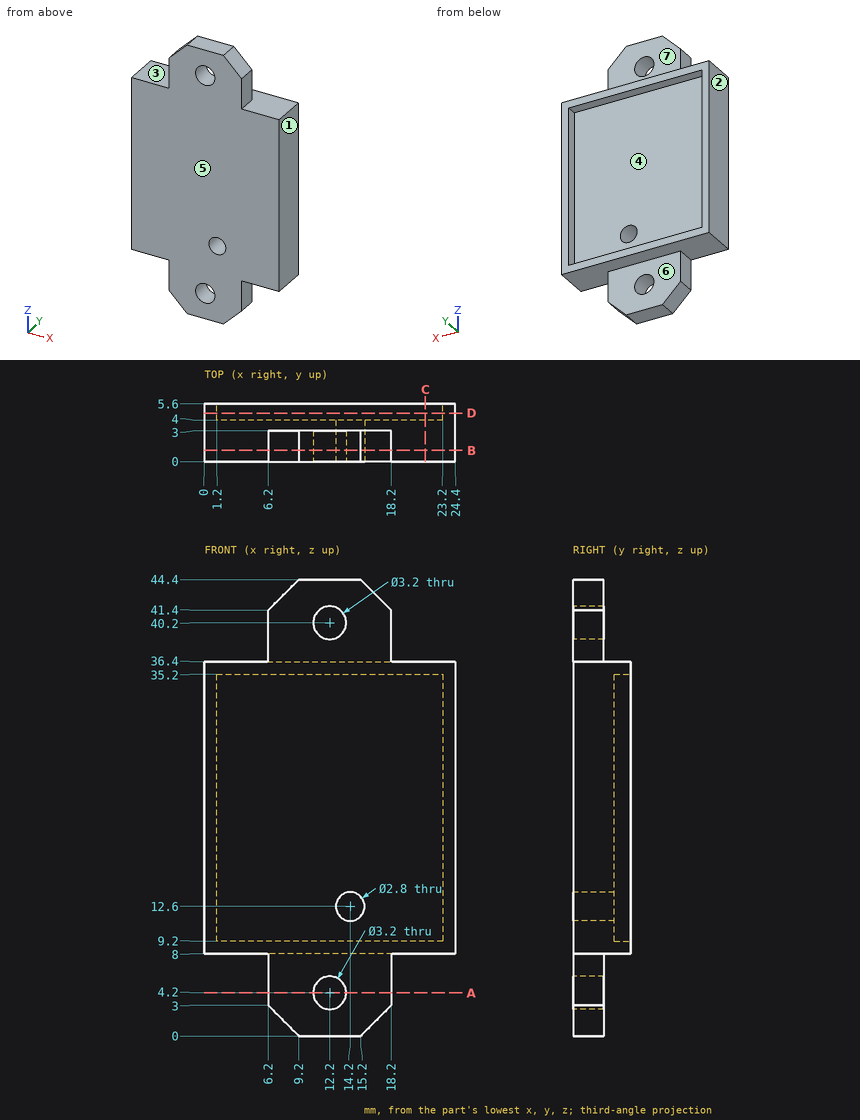
Verification items for this drawing (mm, ordinates from the low corner). A direction names the side the tool comes from. Coordinates: 2 decimals unless noted, no trailing zeros. Order: outer loops, then holes, each group sorted by start corner. A loop starts at its lowest first (then second) coordinate and runs counter-clockwise, first axis right, second up. Notation, with made-up numbers: (-20.75, 58) -> (27.25, 58) arc R22 ccw to (27.25, 73) -> close; hole circle Ø6 at (-27.5, 6.25). An arc over 180 degrees is marked (long way). Put each result on its own line as item: value. Start each with the question number.
1. Access from +Z, -Z, +X, -X, +Y, -Y to the whole of each face (thin tool, end or side, straight path). Record for the marked faces 5, 6 and 7.
2. Mould release check, pull along X, two halves, no side actions. Record for the marked faces 1, 2, 3 and 4: released by +X, released by -X, zero draft, split by the parting line, or undercut.
3. Material ranges on L1, parallel to Z at x = 12.2, y = 1.05; L2, parallel to X at y = 1.5, z = 12.6; L3, parallel to X at y = 2.45, z = 40.2, recorded low to high. Write a range as [from, to].
4. Go/stop test with flat-tipped pins: pin 1 Ø0.9 at (y, z) = (1, 5) entering from +X; pin 2 Ø2.5 at (x, z) = (12.2, 4.2) entering from +Y; pin 3 Ø0.8 at (x, y) = (8.5, 4.5) entering from +Z; pin 4 Ø1.5 at (y, z) = (1.5, 38) entering from -X. Record where each tip stops, or that it passes through.
5. Cross-section at C-C, the plane x = 21.5. Record the boundary of the cut face in (y, z).
6. Cross-section at D-D, the plane y = 4.7. Record the boundary of the cut face in (x, z), then the cut area to 3 significant figures.
7. Cross-section at B-B, the plane y = 1.1. Record the boundary of the cut face in (x, z), then the cut area to 3 significant figures.
8. Cross-section at A-A, the plane z = 4.2. Record the boundary of the cut face in (x, y), then the cut area to 3 significant figures.
Computed:
1. face 5: +Z, -Z, +X, -X, -Y
1. face 6: -Z, +X, -X, +Y
1. face 7: +Z, +X, -X, +Y
2. face 1: released by +X
2. face 2: released by -X
2. face 3: zero draft
2. face 4: undercut
3. L1: [0, 2.6], [5.8, 38.6], [41.8, 44.4]
3. L2: [0, 12.8], [15.6, 24.4]
3. L3: [6.2, 10.6], [13.8, 18.2]
4. pin 1: x = 18.2
4. pin 2: through
4. pin 3: z = 36.4
4. pin 4: x = 6.2
5. outline: (0, 8) -> (5.6, 8) -> (5.6, 9.2) -> (4, 9.2) -> (4, 35.2) -> (5.6, 35.2) -> (5.6, 36.4) -> (0, 36.4) -> close
6. outline: (0, 8) -> (24.4, 8) -> (24.4, 36.4) -> (0, 36.4) -> close; hole (1.2, 9.2) -> (23.2, 9.2) -> (23.2, 35.2) -> (1.2, 35.2) -> close
6. area: 121 mm2
7. outline: (0, 8) -> (6.2, 8) -> (6.2, 3) -> (9.2, 0) -> (15.2, 0) -> (18.2, 3) -> (18.2, 8) -> (24.4, 8) -> (24.4, 36.4) -> (18.2, 36.4) -> (18.2, 41.4) -> (15.2, 44.4) -> (9.2, 44.4) -> (6.2, 41.4) -> (6.2, 36.4) -> (0, 36.4) -> close; hole circle Ø3.2 at (12.2, 4.2); hole circle Ø3.2 at (12.2, 40.2); hole circle Ø2.8 at (14.2, 12.6)
7. area: 845 mm2
8. outline: (6.2, 0) -> (10.6, 0) -> (10.6, 3) -> (6.2, 3) -> close; (13.8, 0) -> (18.2, 0) -> (18.2, 3) -> (13.8, 3) -> close
8. area: 26.4 mm2
